Autodesk Inventor part; units mm, degrees
ref_plane "YZ Plane" through (0, 0, 0) normal (1, 0, 0) x (0, 1, 0)
ref_plane "XZ Plane" through (0, 0, 0) normal (0, 1, 0) x (-1, 0, 0)
ref_plane "XY Plane" through (0, 0, 0) normal (0, 0, 1) x (1, 0, 0)
sketch "Sketch1" plane through (0, 0, 0) normal (0, 1, 0) x (-1, 0, 0)
  line L0 (0, 0) -> (0, 8.89)
  line L1 (0, 0) -> (12.7, 0)
  line L2 (12.7, 0) -> (12.7, 8.89)
  line L3 (12.7, 8.89) -> (0, 8.89)
  line L4 (0, 8.89) -> (0, 72.39)
  line L5 (0, 0) -> (-139.7, 0) construction
  line L6 (12.7, 0) -> (12.7, -50.8)
  line L7 (12.7, -50.8) -> (0, -50.8)
  line L8 (0, -50.8) -> (0, 0)
  line L9 (0, 40.64) -> (-26.416, 40.64) construction
  line L10 (-26.416, 40.64) -> (-39.116, 40.64) construction
  line L11 (-39.116, 40.64) -> (-140.716, 40.64) construction
  line L12 (0, 72.39) -> (12.7, 72.39)
  line L13 (12.7, 72.39) -> (12.7, 8.89)
  dimension "d1" = 8.89
  dimension "d3" = 12.7
  dimension "d4" = 63.5
  dimension "d6" = 139.7
  dimension "d7" = 50.8
  dimension "d8" = 26.416
  dimension "d9" = 12.7
  dimension "d10" = 101.6
  dimension "d13" = 31.75
extrude "Extrusion1" add sketch "Sketch1" along normal blind 50.8
sketch "Sketch2" plane through (-12.7, 0, -50.8) normal (-1, 0, 0) x (0, 0, 1)
  line L0 (123.19, 0) -> (0, 0) construction
  line L1 (0, 0) -> (50.8, 0) construction
  line L2 (50.8, 0) -> (59.69, 0) construction
  line L3 (59.69, 0) -> (123.19, 0) construction
  line L4 (123.19, 0) -> (123.19, 50.8) construction
  line L5 (0, 0) -> (0, 50.8)
  circle A0 centre (49.53, 38.1) radius 1.905
  circle A1 centre (24.13, 12.7) radius 1.905
  circle A2 centre (49.53, 12.7) radius 1.905
  circle A3 centre (49.53, 38.1) radius 4.445
  circle A4 centre (24.13, 12.7) radius 4.445
  circle A5 centre (49.53, 12.7) radius 4.445
  line L6 (0, 25.4) -> (13.335, 25.4)
  line L7 (59.69, 0) -> (59.69, 50.8)
  line L8 (123.19, 50.8) -> (0, 50.8)
  dimension "d16" = 50.8
  dimension "d17" = 63.5
  dimension "d32" = 3.81
  dimension "d34" = 3.81
  dimension "d36" = 3.81
  dimension "d38" = 8.89
  dimension "d39" = 8.89
  dimension "d40" = 8.89
  dimension "d41" = 25.4
  dimension "d42" = 25.4
  dimension "d43" = 10.16
  dimension "d49" = 12.7
  dimension "d50" = 12.7
  dimension "d51" = 12.7
extrude "Extrusion4" cut sketch "Sketch2" against normal through all contours A0 | A1 | A2
extrude "Extrusion5" cut sketch "Sketch2" along normal blind 7.62 from surface at -12.7 contours A0 | A3 | A4 | A5
chamfer "Chamfer1" distance 25.4 angle 45 1 edges at (-6.35, 50.8, -50.8)
fillet "Fillet3" radius 12.7 3 edges at (-6.35, 50.8, -25.4) (-6.35, 25.4, -50.8) (-6.35, 0, -50.8)
fillet "Fillet8" radius 2.54 3 edges at (0, 12.7, -31.115) (0, 12.7, -5.715) (0, 38.1, -5.715)
sketch "Sketch6" plane through (-12.7, 0, 72.39) normal (-1, 0, 0) x (0, 0, 1)
  line L0 (0, 0) -> (0, 50.8)
  line L1 (0, 0) -> (0, 50.8)
  line L2 (0, 25.4) -> (-31.75, 25.4) construction
  circle A0 centre (-31.75, 25.4) radius 7.239
  circle A1 centre (-31.75, 25.4) radius 5.08
  point P0 (-72.39, 0)
  dimension "d87" = 31.75
  dimension "d88" = 14.478
  dimension "d89" = 10.16
extrude "Extrusion11" cut sketch "Sketch6" along normal blind 6.35 from surface at -12.7
extrude "Extrusion12" cut sketch "Sketch6" against normal through all contours A1
sketch "Sketch7" plane through (-12.7, 0, 72.39) normal (-1, 0, 0) x (0, 0, 1)
  circle A0 centre (-31.75, 25.4) radius 7.239 construction
  line L0 (-31.75, 25.4) -> (-31.75, 38.1) construction
  line L1 (-31.75, 25.4) -> (-31.75, 12.7) construction
  circle A1 centre (-31.75, 38.1) radius 1.143
  circle A2 centre (-31.75, 12.7) radius 1.143
  point P0 (-72.39, 0)
  dimension "d95" = 12.7
  dimension "d96" = 12.7
  dimension "d97" = 2.286
  dimension "d98" = 2.286
extrude "Extrusion13" cut sketch "Sketch7" along normal blind 2.54 from surface at -12.7
sketch "Sketch8" plane through (0, 0, 72.39) normal (1, 0, 0) x (0, 0, -1)
  circle A0 centre (31.75, 25.4) radius 5.08
  circle A1 centre (31.75, 25.4) radius 25.4
  line L0 (92.5295, 50.8) -> (0, 50.8)
  line L1 (31.75, 50.8) -> (0, 50.8)
  line L2 (0, 0) -> (0, 50.8)
  line L3 (0, 0) -> (31.75, 0)
  line L4 (110.49, 0) -> (0, 0)
  point P0 (72.39, 0)
extrude "Extrusion14" cut sketch "Sketch8" against normal through all contours A1 L3 L2 L0
sketch "Sketch9" plane through (-12.7, 12.7, -50.8) normal (-1, 0, 0) x (0, 0, 1)
  circle A0 centre (24.13, 0) radius 1.905 construction
  line L0 (24.13, 0) -> (24.13, -12.7) construction
  line L1 (91.44, -12.7) -> (12.7, -12.7) construction
  line L2 (24.13, 0) -> (11.43, 0) construction
  line L3 (11.43, 0) -> (11.43, 24.13)
  line L4 (21.6803, 34.3803) -> (3.7197, 16.4197) construction
  arc A1 (0, 0) -> (12.7, -12.7) centre (12.7, 0) ccw construction
  circle A2 centre (49.53, 0) radius 1.905 construction
  circle A3 centre (24.13, 0) radius 1.905 construction
  circle A4 centre (49.53, 25.4) radius 1.905 construction
  arc A5 (91.44, -12.7) -> (91.44, 38.1) centre (91.44, 12.7) ccw construction
  line L5 (30.6605, 38.1) -> (91.44, 38.1) construction
  arc A6 (30.6605, 38.1) -> (21.6803, 34.3803) centre (30.6605, 25.4) ccw construction
  line L6 (3.7197, 16.4197) -> (21.6803, 34.3803) construction
  arc A7 (3.7197, 16.4197) -> (0, 7.4395) centre (12.7, 7.4395) ccw construction
  line L7 (0, 0) -> (0, 7.4395) construction
  arc A8 (0, 0) -> (12.7, -12.7) centre (12.7, 0) ccw construction
  line L8 (12.7, -12.7) -> (91.44, -12.7) construction
  circle A9 centre (91.44, 12.7) radius 5.08 construction
  line L9 (3.7197, 16.4197) -> (21.6803, 34.3803)
  arc A10 (3.7197, 16.4197) -> (0, 7.4395) centre (12.7, 7.4395) ccw
  arc A11 (0, 0) -> (12.7, -12.7) centre (12.7, 0) ccw
  line L10 (0, 20.1395) -> (0, -8.6122)
  circle A12 centre (49.53, 25.4) radius 1.905
  circle A13 centre (49.53, 25.4) radius 12.7
  circle A14 centre (24.13, 0) radius 6.985
  circle A15 centre (24.13, 0) radius 12.7
  line L11 (15.1497, 8.9803) -> (40.5497, 34.3803)
  arc A16 (30.6605, 38.1) -> (21.6803, 34.3803) centre (30.6605, 25.4) ccw
  line L12 (123.19, 38.1) -> (0, 38.1)
  line L13 (12.7, -12.7) -> (91.44, -12.7)
  line L14 (24.13, -12.7) -> (12.7, -12.7)
  point P0 (50.8, -12.7)
  point P1 (11.43, -12.6363)
  point P2 (0, 7.4395)
  point P3 (49.53, 38.1)
  point P4 (24.13, -12.7)
  dimension "d108" = 12.7
  dimension "d56" = 31.75
  dimension "d57" = 2.286
  dimension "d58" = 8.89
  dimension "d59" = 2.286
  dimension "d60" = 8.89
  dimension "d61" = 2.286
  dimension "d62" = 7.62
  dimension "d63" = 2.286
  dimension "d64" = 7.62
  dimension "d65" = 6.35
  dimension "d66" = 6.35
  dimension "d67" = 6.35
  dimension "d68" = 6.35
  dimension "d69" = 6.35
extrude "Extrusion16" cut sketch "Sketch9" against normal through all contours A15 L13 A11 L10 A10 L9 L3 | L3 L9 A16 L12 A13 L11 A15
fillet "Fillet13" radius 3.175 6 edges at (0, 49.8333, -6.1301) (0, 50.8, 19.685) (0, 25.4, 66.04) (0, 0, 6.985) (0, 7.8399, -38.4033) (0, 34.3803, -22.9503)
fillet "Fillet14" radius 7.62 1 edges at (-12.7, 25.4, 35.56)
sketch "Sketch4" plane through (0, 0, 72.39) normal (1, 0, 0) x (0, 0, -1)
  circle A0 centre (31.75, 25.4) radius 3.175
  circle A1 centre (31.75, 25.4) radius 13.97 construction
  circle A2 centre (31.75, 25.4) radius 19.05
  circle A3 centre (31.75, 25.4) radius 25.4
  line L0 (0, 0) -> (110.49, 0)
  line L1 (31.75, 25.4) -> (45.72, 46.6132)
  line L2 (31.75, 25.4) -> (45.72, 4.1868)
  point P0 (72.39, 0)
  point P1 (42.2275, 9.4901)
  point P2 (42.2275, 41.3099)
  dimension "d77" = 27.94
  dimension "d78" = 38.1
sketch "Sketch5" plane through (0, 0, 72.39) normal (1, 0, 0) x (0, 0, -1)
  arc A0 (31.75, 50.8) -> (31.75, 0) centre (31.75, 25.4) ccw
  line L0 (0, 50.8) -> (31.75, 50.8)
  line L1 (0, 0) -> (0, 50.8)
  line L2 (0, 0) -> (31.75, 0)
  point P0 (72.39, 0)
equation "\"d13\" = 0.5 * d4"
properties part number "bearing_bracket_3DPrint"
Build history of the part. All positions in model axes, mm. A direction names the side the tool comes from. Round coordinates to 2 decimals unless told otherwise and drop trailing zeros. Loops run counter-clockwise (first coordinate to the right, second up) from the corner with the lowest first, then second, coordinate; pieces in that order, holes last. Notation, with made-up numbers: M 29.5,25.25 L 84.5,25.25 A12 cw 84.5,40.25 Z; hole C -29.75,-33 d7. An arc over 180 degrees is marked long. Answer as CSV lines item,"result".
1. Wall check: probe 1 along Y at (x, z) = (-11, -3); probe 2 along Y at (x, z) = (-3.8, -1.27) (3 decimals); probe 3 along Z at (x, y) = (-6, 9). Give the ranges that are in metal, low to high. Write a range as [from, to].
Resolved:
probe 1,"y = [0, 11.9], [13.5, 37.3], [38.9, 50.68]"
probe 2,"y = [0, 8.255], [17.145, 33.655], [42.545, 50.8]"
probe 3,"z = [-38.82, -29.13], [-24.21, -3.73], [1.19, 60.04]"
2. Flat gauge pins, fed straight in: P1, Ø4, axis at x = -7, z = 51.5, coming from the +Y side; P2, Ø1.5, axis at x = -6, y = 36.5, coming from the +Z side; P3, Ø5, axis at x = -3.5, y = 15.5, coming from the -Z side. Where does each tip first touch, or does it go through?
Resolved:
P1,"stops at y = 49.2"
P2,"stops at z = 63.84"
P3,"stops at z = -39.37"
3. Two-plate mould, pull along Z, no slides. Class faces 3 (the flat face through (0, 25, 24)), 4 (the cylindrical face through (-7.871, 25.959, 66.034)), 5 (the cylindrical face through (-5.044, 8.293, -27.249)), 6 (the cylindrical face through (-8, 8.03, -38.48)): released by +Z, released by -Z, zero draft, split by the parting line, or undercut.
Resolved:
face 3,"zero draft"
face 4,"released by +Z"
face 5,"undercut"
face 6,"released by -Z"
4. Cut at A-A on x = -9.5. Write the cut outline in (y, z) (3 decimals).
Resolved:
outline,"M 0,-26.67 A12.7 ccw 21.68,-35.65 L 47.08,-10.25 A12.7 ccw 50.8,-1.27 L 50.8,40.64 A25.4 ccw 0,40.64 Z; hole C 12.7,-26.67 d3.81; hole C 12.7,-1.27 d3.81; hole C 25.4,40.64 d12.773; hole C 38.1,-1.27 d3.81"
5. 3-axis set-ups, long thin cutter, end or side, ignore diameter. For faces 1 (the cylindrical face through (-1.252, 11.928, 39.798)), 2 (the cylindrical face through (-0.95, 0.91, 7.46)): which of +Z, -Z, +X, -X, +Y, -Y reach the whole face in a straight line?
Resolved:
face 1,"+X"
face 2,"+Z, -Z, +X, -Y"
